Read the model definition and answer for the solid it produces. Units are mm, in the model's axes. Coordinates: 2 decimals unless noted, no trailing zeros. Order: outer loops, then holes, each group sorted by start corner. A loop starts at its lowest first (then second) coordinate and runs counter-clockwise, first axis right, second up. Notation, with made-up numbers: M -23,81 L 34,81 A10 cw 34,89 Z; hole C -18,-24.5 d8. An arc over 180 degrees is marked long. Use a Markdown table: item, result. Add a question column.
1) Find the intervals of material crossed by probe 1 along X at (y, z) = (11.5, 3.75); probe 2 along X at (y, z) = (22, 0.5); probe 3 along X at (y, z) = (14, 6.5), in increasing order. Write a range as [from, to].
2) Find section B-B on y = 3.5. Write down the section's boundary in (x, z).
3) Find section A-A on y = 12. Write down the section's boundary in (x, z).
4) Each of these flat-tipped pins is pushed along its axis until it touches: pin 1 Ø12.5 at (x, y) = (-125, 20.2) entering from +Z; pin 2 Ø1.5 at (y, z) = (28, 4) entering from +X; pin 3 Ø1.2 at (y, z) = (20, -3) entering from +X; pin 4 Ø6.5 at (x, y) = (16.5, 20.5) entering from +Z. Where does it stop, or does it pass through?
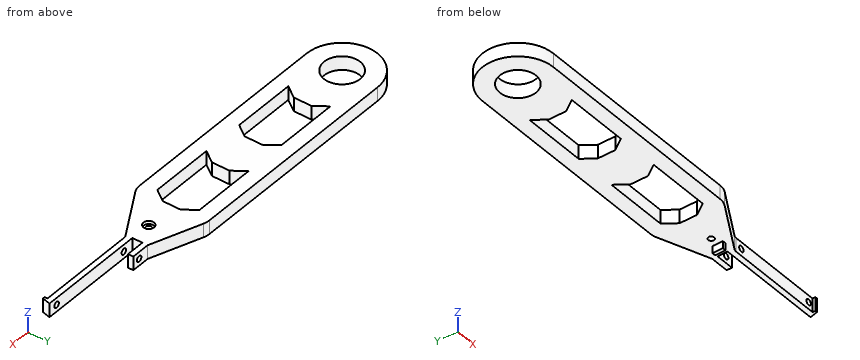
from build123d import *

# Parameters (mm, degrees)
SKETCH_R            = 10.3
PAD_DEPTH           = 7.8
SKETCH001_R         = 1.65
HOLE_DEPTH          = 22.485586
FILLET_R            = 10
FILLET001_R         = 4
HOLE001_D           = 3.3
HOLE001_CBORE_D     = 6
HOLE001_CBORE_DEPTH = 1.8
SKETCH003_W         = 2
SKETCH003_H         = 6
PAD001_DEPTH        = 4


with BuildPart() as part:
    # Sketch → Pad (new body)
    with BuildSketch(Plane.XY):
        with BuildLine():
            ThreePointArc((-125, 40.4), (-145.2, 20.2), (-125, 0))
            Line((-125, 0), (0, 0))
            Line((31.030407, 17.915414), (0, 0))
            Line((31.030407, 17.915414), (88.030407, 17.915414))
            Line((88.030407, 16.315414), (88.030407, 17.915414))
            Line((89.230407, 16.315414), (88.030407, 16.315414))
            Line((90.430407, 20.915414), (89.230407, 16.315414))
            Line((88.030407, 20.915414), (90.430407, 20.915414))
            Line((31.030407, 20.915414), (88.030407, 20.915414))
            Line((29.630407, 20.915414), (31.030407, 20.915414))
            Line((29.630407, 26.615414), (29.630407, 20.915414))
            Line((40.130407, 26.615414), (29.630407, 26.615414))
            Line((40.130407, 29.615414), (40.130407, 26.615414))
            Line((29.630407, 29.615414), (40.130407, 29.615414))
            Line((0, 40.4), (29.630407, 29.615414))
            Line((-125, 40.4), (0, 40.4))
        make_face()
        with Locations((-125, 20.2)):
            Circle(SKETCH_R, mode=Mode.SUBTRACT)
        Polygon((-101, 32.2), (-96, 25.2), (-96, 15.2), (-101, 8.2), (-65, 8.2), (-60, 15.2), (-60, 25.2), (-65, 32.2), align=None, mode=Mode.SUBTRACT)
        Polygon((-41, 32.2), (-36, 25.2), (-36, 15.2), (-41, 8.2), (-5, 8.2), (0, 15.2), (0, 25.2), (-5, 32.2), align=None, mode=Mode.SUBTRACT)
    extrude(amount=PAD_DEPTH)

    # Sketch001 (on Face5 of Pad) → Hole (cut, through all)
    with BuildSketch(Plane.XZ.offset(-17.915414)):
        with Locations((85.180407, 3.9)):
            Circle(SKETCH001_R)
        with Locations((35.880407, 3.9)):
            Circle(SKETCH001_R)
    extrude(amount=-HOLE_DEPTH, mode=Mode.SUBTRACT)

    # Fillet
    fillet_edges = [part.edges().sort_by_distance(p)[0] for p in [
        (0, 0, 3.9),
        (0, 40.4, 3.9),
    ]]
    fillet(fillet_edges, radius=FILLET_R)

    # Fillet001
    fillet001_edges = [part.edges().sort_by_distance(p)[0] for p in [
        (31.030407, 17.915414, 3.9),
    ]]
    fillet(fillet001_edges, radius=FILLET001_R)

    # Hole001 (through all)
    with Locations(Plane.XY.offset(7.8)):
        with Locations((17.630407, 20.915414)):
            CounterBoreHole(HOLE001_D / 2, HOLE001_CBORE_D / 2, HOLE001_CBORE_DEPTH)

    # Sketch003 (on Face1 of Hole001) → Pad001 (join)
    with BuildSketch(Plane(origin=(0, 0, 0), x_dir=(1, 0, 0), z_dir=(0, 0, -1))):
        with Locations((23.280407, -20.915414)):
            Rectangle(SKETCH003_W, SKETCH003_H)
    extrude(amount=PAD001_DEPTH)


solid = part.part
Check result:
| question | item | result |
|---|---|---|
| 1 | probe 1 | x = [-143.23, -130.51], [-119.49, -98.64], [-62.64, -38.64], [-2.64, 19.92] |
| 1 | probe 2 | x = [-145.12, -135.14], [-114.86, -96], [-60, -36], [0, 16.39], [18.87, 29.63] |
| 1 | probe 3 | x = [-144.22, -133.22], [-116.78, -96.86], [-60.86, -36.86], [-0.86, 24.25] |
| 2 | outline | M -136.36,0 L 6.06,0 L 6.06,7.8 L -136.36,7.8 Z |
| 3 | outline | M -143.46,0 L -131.23,0 L -131.23,7.8 L -143.46,7.8 Z; M -118.77,0 L -98.29,0 L -98.29,7.8 L -118.77,7.8 Z; M -62.29,0 L -38.29,0 L -38.29,7.8 L -62.29,7.8 Z; M -2.29,0 L 20.78,0 L 20.78,7.8 L -2.29,7.8 Z |
| 4 | pin 1 | passes through |
| 4 | pin 2 | stops at x = 40.13 |
| 4 | pin 3 | stops at x = 24.28 |
| 4 | pin 4 | stops at z = 7.8 |
